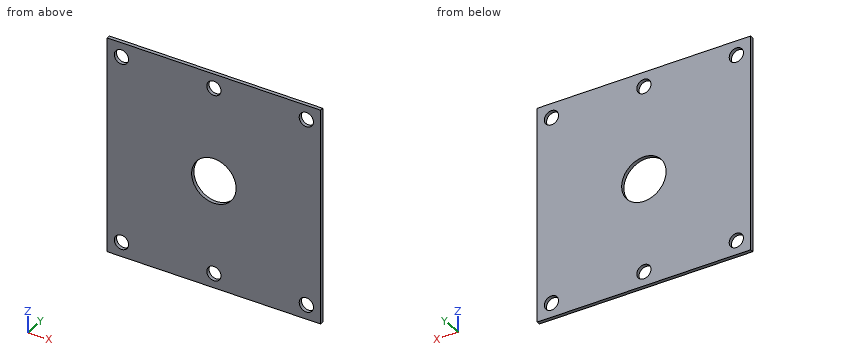
```python
from build123d import *

# Parameters (mm, degrees)
SKETCH1_W           = 60
SKETCH1_H           = 60
BOSS_EXTRUDE1_DEPTH = 1
SKETCH2_R           = 2
CUT_EXTRUDE1_DEPTH  = 2
SKETCH4_R           = 6.25
CUT_EXTRUDE3_DEPTH  = 10


with BuildPart() as part:
    # Sketch1 → Boss-Extrude1 (new body)
    with BuildSketch(Plane(origin=(0, 0, 0), x_dir=(1, 0, 0), z_dir=(0, 1, 0))):
        Rectangle(SKETCH1_W, SKETCH1_H)
    extrude(amount=BOSS_EXTRUDE1_DEPTH)

    # Sketch2 → Cut-Extrude1 (cut, through all)
    with BuildSketch(Plane(origin=(0, 1, 0), x_dir=(1, 0, 0), z_dir=(0, 1, 0))):
        with Locations((-26, 26)):
            Circle(SKETCH2_R)
        with Locations((0, 26)):
            Circle(SKETCH2_R)
        with Locations((26, 26)):
            Circle(SKETCH2_R)
        with Locations((26, -26)):
            Circle(SKETCH2_R)
        with Locations((0, -26)):
            Circle(SKETCH2_R)
        with Locations((-26, -26)):
            Circle(SKETCH2_R)
    extrude(amount=-CUT_EXTRUDE1_DEPTH, mode=Mode.SUBTRACT)

    # Sketch4 → Cut-Extrude3 (cut)
    with BuildSketch(Plane(origin=(0, 1, 0), x_dir=(1, 0, 0), z_dir=(0, 1, 0))):
        Circle(SKETCH4_R)
    extrude(amount=-CUT_EXTRUDE3_DEPTH, mode=Mode.SUBTRACT)


solid = part.part
```
Input: part model. Units: mm. Frame: model coordinates. Coordinates: 2 decimals unless noted, no trailing zeros. Order: outer loops, then holes, each group sorted by start corner. A loop starts at its lowest first (then second) coordinate and runs counter-clockwise, first axis right, second up. Notation, with made-up numbers: (63, 47) - (86, 47) arc R22 ccw to (86, 81) - close; hole circle Ø8 at (65.5, -2). An arc over 180 degrees is marked (long way). Put each result on its own line as item: value.
1. Line query: line 1 along Z through (x, y) = (26, 0.45); line 2 along X through (y, z) = (0.55, 26); line 3 along X through (y, z) = (0.45, 0). Output: solid intervals per line, ascending.
Report:
line 1: z = -30 to -28, -24 to 24, 28 to 30
line 2: x = -30 to -28, -24 to -2, 2 to 24, 28 to 30
line 3: x = -30 to -6.25, 6.25 to 30
2. Cut plane D-D on x = 0. Return the cut outline in (y, z).
Report:
outline: (0, -30) - (1, -30) - (1, -28) - (0, -28) - close; (0, -24) - (1, -24) - (1, -6.25) - (0, -6.25) - close; (0, 6.25) - (1, 6.25) - (1, 24) - (0, 24) - close; (0, 28) - (1, 28) - (1, 30) - (0, 30) - close
3. Cut plane B-B on x = -26. Return the cut outline in (y, z), then the cut area to 3 significant figures.
Report:
outline: (0, -30) - (1, -30) - (1, -28) - (0, -28) - close; (0, -24) - (1, -24) - (1, 24) - (0, 24) - close; (0, 28) - (1, 28) - (1, 30) - (0, 30) - close
area: 52.0 mm2
4. Contact query for a flat-ended pin moving along its axis: pin 1 Ø1 at (x, z) = (21.5, 23.5) entering from -Y. Output: stop coordinate, or through.
Report:
pin 1: stops at y = 0
5. Cut plane C-C on z = 0. Return the cut outline in (x, y), then the cut area to 3 significant figures.
Report:
outline: (-30, 0) - (-6.25, 0) - (-6.25, 1) - (-30, 1) - close; (6.25, 0) - (30, 0) - (30, 1) - (6.25, 1) - close
area: 47.5 mm2
6. Cut plane A-A on z = 26. Return the cut outline in (x, y), then the cut area to 3 significant figures.
Report:
outline: (-30, 0) - (-28, 0) - (-28, 1) - (-30, 1) - close; (-24, 0) - (-2, 0) - (-2, 1) - (-24, 1) - close; (2, 0) - (24, 0) - (24, 1) - (2, 1) - close; (28, 0) - (30, 0) - (30, 1) - (28, 1) - close
area: 48.0 mm2
